```python
from build123d import *

# Parameters (mm, degrees)
SKETCH1_R           = 5
SKETCH1_R_2         = 2.5
BOSS_EXTRUDE1_DEPTH = 7.25
SKETCH5_R           = 12.5
SKETCH5_R_2         = 6
CUT_EXTRUDE1_DEPTH  = 58.063561053
CIRPATTERN1_COUNT   = 4
SKETCH6_R           = 1.25
CUT_EXTRUDE2_DEPTH  = 10


with BuildPart() as part:
    # Sketch1 → Boss-Extrude1 (new, symmetric)
    with BuildSketch(Plane(origin=(0, 0, 0), x_dir=(0, 0, -1), z_dir=(1, 0, 0))):
        with Locations(Location((0, 0, 0), (0, 0, 180))):
            Circle(SKETCH1_R)
        with Locations(Location((0, 0, 0), (0, 0, 180))):
            Circle(SKETCH1_R_2, mode=Mode.SUBTRACT)
    extrude(amount=BOSS_EXTRUDE1_DEPTH, both=True)

    # Sketch4 → Revolve4 (revolve)
    with BuildSketch(Plane.XY, mode=Mode.PRIVATE) as revolve4_sk:
        Polygon((-4.75, 5), (-4.75, 35), (-7.25, 35), (-7.25, 40), (2.75, 40), (2.75, 35), (0.25, 35), (0.25, 5), align=None)
    revolve(revolve4_sk.sketch.rotate(Axis((0, 0, 0), (-1, 0, 0)), 90), axis=Axis((0, 0, 0), (-1, 0, 0)))

    # Sketch5 → Cut-Extrude1 (cut, symmetric)
    with BuildSketch(Plane(origin=(0.25, 0, 0), x_dir=(0, 0, -1), z_dir=(1, 0, 0))):
        with Locations((0, 20)):
            Circle(SKETCH5_R)
        with Locations((-19.445436483, 19.445436483)):
            Circle(SKETCH5_R_2)
    cut_extrude1 = extrude(amount=CUT_EXTRUDE1_DEPTH, both=True, mode=Mode.SUBTRACT)

    # CirPattern1: Cut-Extrude1 ×4 about axis
    cirpattern1_axis = Axis((0, 0, 0), (1, 0, 0))
    for i in range(1, CIRPATTERN1_COUNT):
        add(cut_extrude1.rotate(cirpattern1_axis, i * 360 / CIRPATTERN1_COUNT), mode=Mode.SUBTRACT)

    # Sketch6 → Cut-Extrude2 (cut, symmetric)
    with BuildSketch(Plane.XY):
        with Locations((3.75, 0)):
            Circle(SKETCH6_R)
    extrude(amount=CUT_EXTRUDE2_DEPTH, both=True, mode=Mode.SUBTRACT)


solid = part.part
```
For this review, take the finished solid that the model builds, in its own axes (mm). A direction names the side the tool comes from. Coordinates: 2 decimals unless noted, no trailing zeros. Loops run counter-clockwise (first coordinate to the right, second up) from the corner with the lowest first, then second, coordinate; pieces in that order, holes last. Notation, with made-up numbers: (50, 22.5) - (108, 22.5) arc R18 ccw to (108, 52.5) - close; hole circle Ø2 at (51, -4). An arc over 180 degrees is marked (long way). Use one line per item in the form item = value. Start each with the question number.
1) Draft analysis for pull direction Z (two halves, no side actions). For faces 1 (the face through (-2.18, -1.76, 39.96)), 2 (the face through (-6.018, 34.168, 7.587)), 3 (the face through (7.25, 2, 2)), state which applies: released by +Z, released by -Z, zero draft, split by the parting line, or undercut.
2) Take a section at A-A (z = 0). State how many separate pieces and enclosed holes the cut face has, plus the area to 4 significant figures.
3) Take a section at D-D (x = 3.75). State the section outline as (y, z) points.
4) For pin 1 (5 mm diameter, centred on y = -14, z = -31, fed in from +X); pin 2 (3 mm diameter, centred on x = -1, z = -8, fed in from -Y); pin 3 (21 mm diameter, centred on y = -15.5, z = -10, fed in from +X), all flat-tipped, find the tip position at first contact; note any pin that passes through.
5) Take a section at B-B (y = -18). State the section outline as (x, z) points, plus the area to 3 significant figures.
6) To check wall thickness, follow probe 1 along Y at (x, z) = (-3.45, 0); probe 2 along Y at (x, z) = (1.7, 0); probe 3 along Z at (x, y) = (2, -3.5). State the ranges of each line that lie inside material, in increasing order. Write a range as from..to.
7) For faces 4 (the face through (1.482, 34.168, 7.587)), 5 (the face through (-4.75, 5, 2)), 6 (the face through (-2.22, -8.91, 5.77)), list the 3-axis set-ups (+Z, -Z, +X, -X, +Y, -Y) from which the entire face can be reached by the end or side of a thin tool; tool diameter is ignored.
8) Take a section at C-C (y = -27). State the section outline as (x, z) points, plus the area to 3 significant figures.
From the geometry:
q1.face_1 = split by the parting line
q1.face_2 = undercut
q1.face_3 = zero draft
q2.separate_pieces = 4
q2.enclosed_holes = 0
q2.area = 222.5 mm2
q3.outline = (-1.25, -4.84) - (-1.25, -2.17) arc R2.5 cw to (-1.25, 2.17) - (-1.25, 4.84) arc R5 ccw to start; (1.25, -4.84) arc R5 ccw to (1.25, 4.84) - (1.25, 2.17) arc R2.5 cw to (1.25, -2.17) - close
q4.pin_1 = 2.75
q4.pin_2 = -39.47
q4.pin_3 = 0.25
q5.outline = (-7.25, -35.72) - (2.75, -35.72) - (2.75, -30.02) - (0.25, -30.02) - (0.25, -25.27) - (-4.75, -25.27) - (-4.75, -30.02) - (-7.25, -30.02) - close; (-7.25, 30.02) - (-4.75, 30.02) - (-4.75, 25.27) - (0.25, 25.27) - (0.25, 30.02) - (2.75, 30.02) - (2.75, 35.72) - (-7.25, 35.72) - close; (-4.75, -13.62) - (0.25, -13.62) - (0.25, -12.34) - (-4.75, -12.34) - close; (-4.75, 12.34) - (0.25, 12.34) - (0.25, 13.62) - (-4.75, 13.62) - close
q5.area = 174 mm2
q6.probe_1 = -40..-32.5, -7.5..-2.5, 2.5..7.5, 32.5..40
q6.probe_2 = -40..-35, -5..-2.5, 2.5..5, 35..40
q6.probe_3 = -39.85..-34.82, -3.57..3.57, 34.82..39.85
q7.face_4 = +X
q7.face_5 = -X
q7.face_6 = +X, -X
q8.outline = (-7.25, -29.51) - (2.75, -29.51) - (2.75, -22.27) - (0.25, -22.27) - (0.25, -10.36) - (-4.75, -10.36) - (-4.75, -22.27) - (-7.25, -22.27) - close; (-7.25, 22.27) - (-4.75, 22.27) - (-4.75, 10.36) - (0.25, 10.36) - (0.25, 22.27) - (2.75, 22.27) - (2.75, 29.51) - (-7.25, 29.51) - close
q8.area = 264 mm2
